Input: part model. Units: mm. Frame: model coordinates. Face numbers are marked on the shaded views. Give positions to 0.01 mm unless a question says otherwise; leave off trailing zeros. Write each loop counter-clockwise with the first axis right and the second up, starting at its lowest first coordinate (ties: lowest second). Pieces come first, ordered by that corner, then holes. Notation, with made-up numbers: (-6.75, 28.25) - (18.25, 28.25) arc R32 cw to (18.25, 58.25) - close; hole circle Ø8 at (24, 67). An arc over 180 degrees is marked (long way). Answer as CSV lines item,"result".
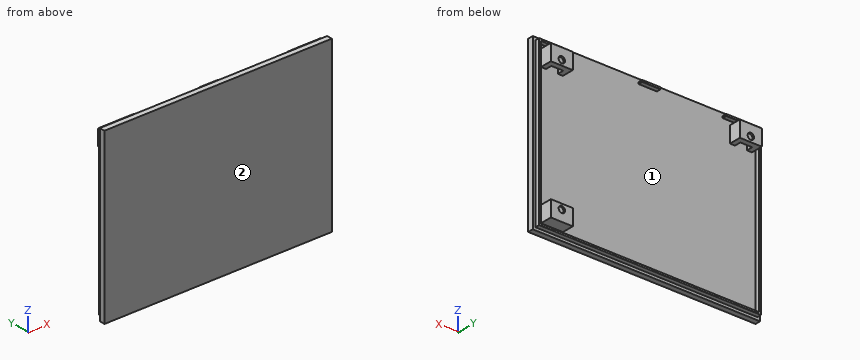
```python
from build123d import *

# Parameters (mm, degrees)
SKETCH_1_W          = 124.5
SKETCH_1_H          = 93
EXTRUDE_1_DEPTH     = 3
SKETCH_2_W          = 10
SKETCH_2_H          = 1
EXTRUDE_1_2_DEPTH   = 2.4
EXTRUDE_2_DEPTH     = 3.5
SKETCH_4_W          = 12
SKETCH_4_H          = 8.814582562
EXTRUDE_3_DEPTH     = 3
SKETCH_5_R          = 1.75
CUT_EXTRUDE_1_DEPTH = 1


with BuildPart() as part:
    # Эскиз1 → Extrude 1 (new body)
    with BuildSketch(Plane(origin=(0, 0, 0), x_dir=(1, 0, 0), z_dir=(0, 1, 0))):
        Rectangle(SKETCH_1_W, SKETCH_1_H)
    extrude(amount=EXTRUDE_1_DEPTH)

    # Эскиз2 → Extrude 1 2 (add)
    with BuildSketch(Plane(origin=(0, 3, 0), x_dir=(1, 0, 0), z_dir=(0, 1, 0))):
        Polygon((-41.75, -44), (-59.75, -44), (-59.75, 44), (59.75, 44), (59.75, -44), (47.25, -44), (47.25, -45), (60.75, -45), (60.75, 45), (-60.75, 45), (-60.75, -45), (-41.75, -45), align=None)
        with Locations((-0.75, -44.5)):
            Rectangle(SKETCH_2_W, SKETCH_2_H)
    extrude(amount=EXTRUDE_1_2_DEPTH)

    # Эскиз3 → Бобышка-Вытянуть2 (add)
    with BuildSketch(Plane(origin=(0, 3, 0), x_dir=(1, 0, 0), z_dir=(0, 1, 0))):
        Polygon((-55, -36), (-55, -33.185417438), (-57.75, -33.185417438), (-57.75, -42), (-45.75, -42), (-45.75, -33.185417438), (-48.5, -33.185417438), (-48.5, -36), (-50.125, -38.814582562), (-53.375, -38.814582562), align=None)
        Polygon((55, 36), (55, 33.185417438), (57.75, 33.185417438), (57.75, 42), (45.75, 42), (45.75, 33.185417438), (48.5, 33.185417438), (48.5, 36), (50.125, 38.814582562), (53.375, 38.814582562), align=None)
        Polygon((55, -36), (55, -33.185417438), (57.75, -33.185417438), (57.75, -42), (45.75, -42), (45.75, -33.185417438), (48.5, -33.185417438), (48.5, -36), (50.125, -38.814582562), (53.375, -38.814582562), align=None)
    extrude(amount=EXTRUDE_2_DEPTH)

    # Эскиз4 → Бобышка-Вытянуть3 (add)
    with BuildSketch(Plane(origin=(0, 6.5, 0), x_dir=(1, 0, 0), z_dir=(0, 1, 0))):
        with Locations((-51.75, -37.592708719)):
            Rectangle(SKETCH_4_W, SKETCH_4_H)
        with Locations((51.75, -37.592708719)):
            Rectangle(SKETCH_4_W, SKETCH_4_H)
        with Locations((51.75, 37.592708719)):
            Rectangle(SKETCH_4_W, SKETCH_4_H)
    extrude(amount=EXTRUDE_3_DEPTH)

    # Эскиз5 → Вырез-Вытянуть1 (cut)
    with BuildSketch(Plane(origin=(0, 9.5, 0), x_dir=(1, 0, 0), z_dir=(0, 1, 0))):
        with Locations(Location((-51.75, -36, 0), (0, 0, 270))):
            Circle(SKETCH_5_R)
        with Locations(Location((51.75, -36, 0), (0, 0, 270))):
            Circle(SKETCH_5_R)
        with Locations(Location((51.75, 36, 0), (0, 0, 270))):
            Circle(SKETCH_5_R)
    extrude(amount=-CUT_EXTRUDE_1_DEPTH, mode=Mode.SUBTRACT)


solid = part.part
```
Item 1: Cut plane A-A on x = 30. Return the cut outline in (y, z).
The answers:
outline,"(0, -46.5) - (3, -46.5) - (3, -45) - (5.4, -45) - (5.4, -44) - (3, -44) - (3, 46.5) - (0, 46.5) - close"
Item 2: Cut plane B-B on z = 1.5. Return the cut outline in (x, y), plus the area to 3 significant figures.
The answers:
outline,"(-62.25, 0) - (62.25, 0) - (62.25, 3) - (60.75, 3) - (60.75, 5.4) - (59.75, 5.4) - (59.75, 3) - (-59.75, 3) - (-59.75, 5.4) - (-60.75, 5.4) - (-60.75, 3) - (-62.25, 3) - close"
area,"378 mm²"
Item 3: Ray query, line 1 (X direction, y = 9.1, z = 36); line 2 (X direction, y = 3.5, z = 33); line 3 (X direction, y = 8.95, z = -36). Return the intervals inside material, ascending. Write a range as from..to.
The answers:
line 1,"-57.75..-53.5, -50..-45.75, 45.75..50, 53.5..57.75"
line 2,"-60.75..-59.75, 59.75..60.75"
line 3,"45.75..50, 53.5..57.75"
Item 4: Contact query for flat-ended pins moving along their axis: pin 1 (2.5 mm diameter, centred on x = -47, y = 4.5, fed in from +Z); pin 2 (0.5 mm diameter, centred on y = 4, z = 44.5, fed in from +X); pin 3 (2 mm diameter, centred on x = -52.5, y = 7, fed in from -Z). Output: stop coordinate, or through.
The answers:
pin 1,"z = 45"
pin 2,"x = 60.75"
pin 3,"z = 33.19"
Item 5: Cut plane D-D on x = -51.75. Return the cut outline in (y, z).
The answers:
outline,"(0, -46.5) - (3, -46.5) - (3, -45) - (5.4, -45) - (5.4, -44) - (3, -44) - (3, 38.81) - (6.5, 38.81) - (6.5, 33.19) - (9.5, 33.19) - (9.5, 34.25) - (8.5, 34.25) - (8.5, 37.75) - (9.5, 37.75) - (9.5, 42) - (3, 42) - (3, 44) - (5.4, 44) - (5.4, 45) - (3, 45) - (3, 46.5) - (0, 46.5) - close"
Item 6: Mould query, pull axis Z, two halves, no side actions, for the marked faces 1 and 2. Classes: +Z half, -Z half, draft (parallel to the pull), parting line (faces both ways), or undercut.
The answers:
face 1,"undercut"
face 2,"draft"
